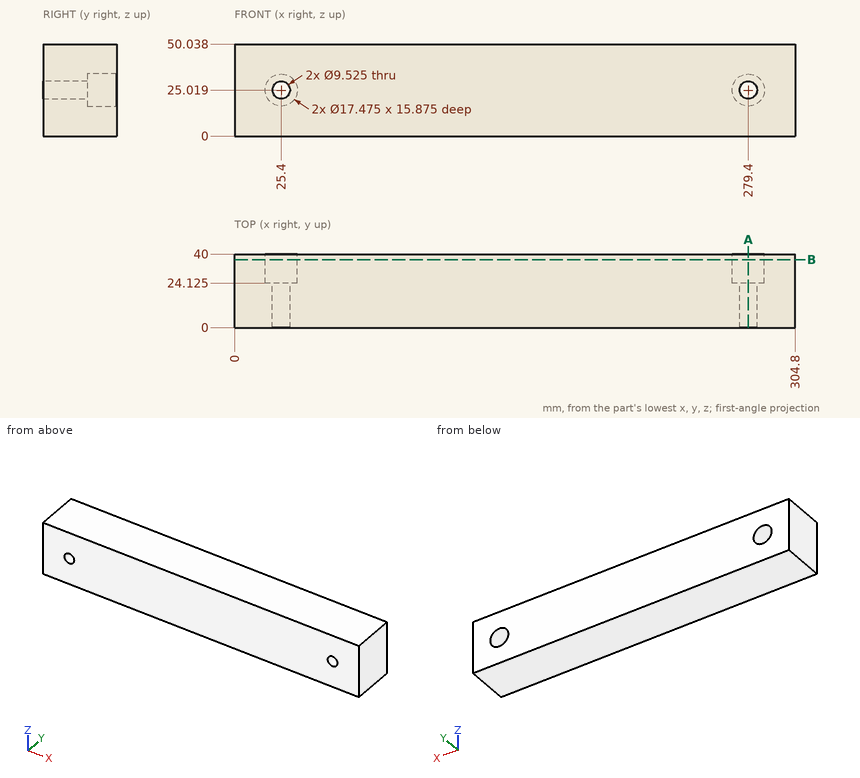
The figure shows three views and two pictorial views of one solid part (mm, origin at its lowest corner). Answer the questions. Give positions to 0.01 mm unless a question says otherwise; leave off trailing zeros. Loops run counter-clockwise (first coordinate to the right, second up) from the corner with the lowest first, then second, coordinate; pieces in that order, holes last. Notation, with made-up numbers: (42.5, 37) - (60.5, 37) arc R15 ccw to (60.5, 56) - close; hole circle Ø6 at (-40, 52.25). An arc over 180 degrees is marked (long way). Answer in a Markdown table with one row per item.
(1) Flat-ended cylindrical pins translate along their axes: pin 1 Ø12 at (x, z) = (247, 14.5) entering from -Y; pin 2 Ø11 at (x, z) = (25.4, 25.019) entering from +Y (3 decimals); pin 3 Ø5.5 at (x, z) = (279.4, 25.019) entering from +Y. Find the tip coordinate at first contact, or state that the pin passes through.
Results list:
| item | result |
|---|---|
| pin 1 | stops at y = 0 |
| pin 2 | stops at y = 24.125 |
| pin 3 | passes through |
(2) Section A-A (x = 279.4) is taken. Give the vertices of the cut face in (y, z) (1 decimal), and give its area (3 significant figures).
Results list:
| item | result |
|---|---|
| outline | (0, 0) - (40, 0) - (40, 16.3) - (24.1, 16.3) - (24.1, 20.3) - (0, 20.3) - close; (0, 29.8) - (24.1, 29.8) - (24.1, 33.8) - (40, 33.8) - (40, 50) - (0, 50) - close |
| area | 1,490 mm² |
(3) Consider L1, parallel to X at y = 25, z = 24; L2, parallel to X at y = 31, z = 18 (1 decimal); L3, parallel to Z at x = 279, y = 13 (1 decimal). Determine where each line is inside the solid, lowest interval first. Write a range as [from, to].
Results list:
| item | result |
|---|---|
| L1 | x = [0, 16.72], [34.08, 270.72], [288.08, 304.8] |
| L2 | x = [0, 20.2], [30.6, 274.2], [284.6, 304.8] |
| L3 | z = [0, 20.3], [29.8, 50] |
(4) Section B-B (y = 37) is taken. Give the vertices of the cut face in (x, z) (1 decimal).
Results list:
| item | result |
|---|---|
| outline | (0, 0) - (304.8, 0) - (304.8, 50) - (0, 50) - close; hole circle Ø17.5 at (25.4, 25); hole circle Ø17.5 at (279.4, 25) |
